The model under review builds one solid part; all positions refer to its coordinate system, in mm. A direction names the side the tool comes from. Coordinates: 2 decimals unless noted, no trailing zeros. Order: outer loops, then holes, each group sorted by start corner. A loop starts at its lowest first (then second) coordinate and runs counter-clockwise, first axis right, second up. Notation, with made-up numbers: M -15,-37.75 L 3,-37.75 A21 ccw 3,-8.75 Z; hole C 81,62 d6. An arc over 180 degrees is marked long. Answer in a Markdown table with one row per item.
from build123d import *

# Parameters (mm, degrees)
SKETCH1_R             = 75
BOSS_EXTRUDE1_DEPTH   = 8
M5X0_8_TAPPED_HOLE1_D = 4.2
SKETCH11_R            = 50.2
CUT_EXTRUDE3_DEPTH    = 6
SKETCH12_R            = 58.6475
SKETCH12_R_2          = 53.6575
CUT_EXTRUDE4_DEPTH    = 4
SKETCH13_R            = 15
CUT_EXTRUDE5_DEPTH    = 2


with BuildPart() as part:
    # Sketch1 → Boss-Extrude1 (new body)
    with BuildSketch(Plane.XY):
        Circle(SKETCH1_R)
    extrude(amount=BOSS_EXTRUDE1_DEPTH)

    # M5x0.8 Tapped Hole1 (through all)
    with Locations(Plane(origin=(0, 0, 0), x_dir=(-1, 0, 0), z_dir=(0, 0, -1))):
        with Locations((-17.470285544, -65.199993275), (-47.72970773, 47.72970773), (65.199993275, -17.470285544), (47.72970773, -47.72970773), (-65.199993275, 17.470285544), (-17.470285544, 65.199993275), (-65.199993275, -17.470285544), (-47.72970773, -47.72970773), (17.470285544, -65.199993275), (65.199993275, 17.470285544), (47.72970773, 47.72970773), (17.470285544, 65.199993275)):
            Hole(M5X0_8_TAPPED_HOLE1_D / 2)

    # Sketch11 → Cut-Extrude3 (cut)
    with BuildSketch(Plane(origin=(0, 0, 0), x_dir=(-1, 0, 0), z_dir=(0, 0, -1))):
        Circle(SKETCH11_R)
    extrude(amount=-CUT_EXTRUDE3_DEPTH, mode=Mode.SUBTRACT)

    # Sketch12 → Cut-Extrude4 (cut)
    with BuildSketch(Plane(origin=(0, 0, 0), x_dir=(-1, 0, 0), z_dir=(0, 0, -1))):
        Circle(SKETCH12_R)
        Circle(SKETCH12_R_2, mode=Mode.SUBTRACT)
    extrude(amount=-CUT_EXTRUDE4_DEPTH, mode=Mode.SUBTRACT)

    # Sketch13 → Cut-Extrude5 (cut)
    with BuildSketch(Plane(origin=(0, 0, 6), x_dir=(-1, 0, 0), z_dir=(0, 0, -1))):
        Circle(SKETCH13_R)
    extrude(amount=-CUT_EXTRUDE5_DEPTH, mode=Mode.SUBTRACT)


solid = part.part
(1) Take a section at C-C (z = 2.75). State how many separate pieces and enclosed holes the cut face has, then the cut area to 3 significant figures.
Report:
| item | result |
|---|---|
| separate pieces | 2 |
| enclosed holes | 14 |
| area | 7,830 mm^2 |
(2) Take a section at D-D (y = 25). Write out the cut boundary in (x, z), then the cut area to 3 significant figures.
Report:
| item | result |
|---|---|
| outline | M -70.71,0 L -53.05,0 L -53.05,4 L -47.48,4 L -47.48,0 L -43.53,0 L -43.53,6 L 43.53,6 L 43.53,0 L 47.48,0 L 47.48,4 L 53.05,4 L 53.05,0 L 70.71,0 L 70.71,8 L -70.71,8 Z |
| area | 564 mm^2 |
(3) Take a section at A-A (y = 0). Write out the cut boundary in (x, z), then the cut area to 3 significant figures.
Report:
| item | result |
|---|---|
| outline | M -75,0 L -58.65,0 L -58.65,4 L -53.66,4 L -53.66,0 L -50.2,0 L -50.2,6 L -15,6 L -15,8 L -75,8 Z; M 15,6 L 50.2,6 L 50.2,0 L 53.66,0 L 53.66,4 L 58.65,4 L 58.65,0 L 75,0 L 75,8 L 15,8 Z |
| area | 498 mm^2 |
(4) The part is to be moulded in two halves that separate along Y. For faces 3 (the flat face through (-1, 18, 8)), 4 (the cylindrical face through (49.67, -48.53, 4.06)), 5 (the cylindrical face through (-9.764, 74.362, 3.944)), say which applies: +Y half, -Y half, draft (parallel to the pull), parting line (faces both ways), or undercut.
Report:
| item | result |
|---|---|
| face 3 | draft |
| face 4 | undercut |
| face 5 | parting line |
(5) Machinability: for faces 1 (the cylindrical face through (18.439, 63.337, 4.056)), 2 (the cylindrical face through (-46.37, -19.23, 2.96)), which of the approach directions +Z, -Z, +X, -X, +Y, -Y give a long, thin tool a straight path to every point of the face, cutting with its end or side? Answer none if there is none.
Report:
| item | result |
|---|---|
| face 1 | +Z, -Z |
| face 2 | -Z |
(6) To check wall thickness, follow line 1 (Y direction, x = 0, z = 7.1); line 2 (X direction, y = 10, z = 1); line 3 (Y direction, x = 17, z = 7.25). State the ranges of each line that lie inside material, in increasing order. Write a range as [from, to].
Report:
| item | result |
|---|---|
| line 1 | [-75, -15], [15, 75] |
| line 2 | [-74.33, -57.79], [-52.72, -49.19], [49.19, 52.72], [57.79, 74.33] |
| line 3 | [-73.05, -67.25], [-63.15, 63.15], [67.25, 73.05] |
(7) Insertion check: P1, Ø3, axis at y = -2.5, z = 4, coming from the +X side; P2, Ø2, axis at x = -11, z = 1.5, coming from the +Y side; P3, Ø6.5, axis at x = 47.73, y = 47.73, coming from the -Z side; P4, Ø1, axis at x = 16, y = -28, coming from the -Z side. Each pin has a flat end and moves straight along its axis. Give the tip position at first contact, or say it passes through.
Report:
| item | result |
|---|---|
| P1 | x = 74.99 |
| P2 | y = 74.33 |
| P3 | z = 0 |
| P4 | z = 6 |
